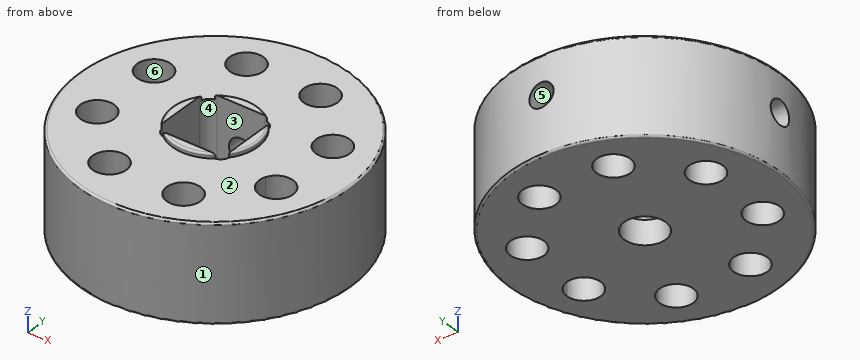
```python
from build123d import *

# Parameters (mm, degrees)
F0_R          = 14
F1_DEPTH      = 10
F2_R          = 4.4
F3_DEPTH      = 0.5
F4_W          = 7
F4_H          = 7
F5_DEPTH      = 8
F6_R          = 2.15
F7_DEPTH      = 2.5
F8_R          = 1.75
F9_DEPTH      = 10
F10_R         = 1.25
F11_DEPTH     = 25
F12_R         = 1.25
F13_DEPTH     = 25
F14_T1_DEPTH  = 10
F14_T6_DEPTH  = 12.5
F14_S7_R      = 4.4
F14_T8_DEPTH  = 8
F14_T13_DEPTH = 12.5
F14_S14_R     = 4.4
F14_T15_DEPTH = 8
F14_T20_DEPTH = 12.5
F14_S21_R     = 4.4
F14_T22_DEPTH = 8
F14_T27_DEPTH = 12.5
F14_S28_R     = 4.4
F14_T29_DEPTH = 8
F15_R         = 0.2


# Not quite as in the source:
# - a fillet or chamfer that OpenCascade refuses, or shapes differently, is made with other operations: its cross-section is extruded or revolved along the edge and cut away or added
# - a feature names something its author has since deleted; it is built from what else it names


with BuildPart() as f1:
    # F0 (on Top) → F1 (new body)
    with BuildSketch(Plane.XY):
        Circle(F0_R)
    extrude(amount=F1_DEPTH)

    # F2 (on face) → F3 (join)
    with BuildSketch(Plane.XY.offset(10)):
        Circle(F2_R)
    extrude(amount=F3_DEPTH)

    # F4 (on face) → F5 (cut)
    with BuildSketch(Plane.XY.offset(10.5)):
        Rectangle(F4_W, F4_H)
    extrude(amount=-F5_DEPTH, mode=Mode.SUBTRACT)

    # F6 (on face) → F7 (cut, through all)
    with BuildSketch(Plane(origin=(0, 0, 0), x_dir=(1, 0, 0), z_dir=(0, 0, -1))):
        Circle(F6_R)
    extrude(amount=-F7_DEPTH, mode=Mode.SUBTRACT)

    # F8 (on face) → F9 (cut, through all)
    with BuildSketch(Plane(origin=(0, 0, 0), x_dir=(1, 0, 0), z_dir=(0, 0, -1))):
        with BuildLine():
            ThreePointArc((7.6220061432, 3.157138317), (9.5802033886, 2.1104600829), (10.9887953251, 3.8268343237))
            ThreePointArc((10.9887953251, 3.8268343237), (8.8973872616, 5.5432085644), (7.6220061432, 3.157138317))
        make_face()
        with Locations((3.8268343237, 9.2387953251)):
            Circle(F8_R)
        with Locations((-3.8268343237, 9.2387953251)):
            Circle(F8_R)
        with Locations((-9.2387953251, 3.8268343237)):
            Circle(F8_R)
        with Locations((-9.2387953251, -3.8268343237)):
            Circle(F8_R)
        with Locations((-3.8268343237, -9.2387953251)):
            Circle(F8_R)
        with Locations((3.8268343237, -9.2387953251)):
            Circle(F8_R)
        with Locations((9.2387953251, -3.8268343237)):
            Circle(F8_R)
    extrude(amount=-F9_DEPTH, mode=Mode.SUBTRACT)

    # F10 (on Front) → F11 (cut)
    with BuildSketch(Plane.XZ):
        with Locations((0, 6)):
            Circle(F10_R)
    extrude(amount=-F11_DEPTH, mode=Mode.SUBTRACT)

    # F12 (on Right) → F13 (cut)
    with BuildSketch(Plane.YZ):
        with Locations((0, 6)):
            Circle(F12_R)
    extrude(amount=-F13_DEPTH, mode=Mode.SUBTRACT)

    # F14: fillet of radius 1 on 4 edges, made by hand

    # F14_s2 → F14_t1 (join)
    with BuildSketch(Plane.XY):
        with BuildLine():
            ThreePointArc((-2.5, -3.5), (-3.2071067812, -3.2071067812), (-3.5, -2.5))
            Line((-3.5, -2.5), (-3.5, -3.5))
            Line((-3.5, -3.5), (-2.5, -3.5))
        make_face()
        with BuildLine():
            ThreePointArc((3.5, -2.5), (3.2071067812, -3.2071067812), (2.5, -3.5))
            Line((2.5, -3.5), (3.5, -3.5))
            Line((3.5, -3.5), (3.5, -2.5))
        make_face()
        with BuildLine():
            ThreePointArc((3.5, 2.5), (3.2071067812, 3.2071067812), (2.5, 3.5))
            Line((2.5, 3.5), (3.5, 3.5))
            Line((3.5, 3.5), (3.5, 2.5))
        make_face()
        with BuildLine():
            ThreePointArc((-2.5, 3.5), (-3.2071067812, 3.2071067812), (-3.5, 2.5))
            Line((-3.5, 2.5), (-3.5, 3.5))
            Line((-3.5, 3.5), (-2.5, 3.5))
        make_face()
    extrude(amount=F14_T1_DEPTH)


with BuildPart() as f14_tool4:
    # F14_s5 → F14_t6 (new body)
    with BuildSketch(Plane.XY.offset(12.5)):
        with BuildLine():
            ThreePointArc((-2.5, -3.5), (-3.2071067812, -3.2071067812), (-3.5, -2.5))
            Line((-3.5, -2.5), (-3.5, -3.5))
            Line((-3.5, -3.5), (-2.5, -3.5))
        make_face()
    extrude(amount=-F14_T6_DEPTH)

    # F14_s7 → F14_t8 (intersect, symmetric)
    with BuildSketch(Plane.XY.offset(6.2)):
        Circle(F14_S7_R)
    extrude(amount=F14_T8_DEPTH, both=True, mode=Mode.INTERSECT)

    split(bisect_by=Plane.XY.offset(10.5), keep=Keep.BOTTOM)


with BuildPart() as f1_1:
    add(f1.part)

    # F14_t3: union F14_tool4
    add(f14_tool4.part)


with BuildPart() as f14_tool11:
    # F14_s12 → F14_t13 (new body)
    with BuildSketch(Plane.XY.offset(12.5)):
        with BuildLine():
            ThreePointArc((3.5, -2.5), (3.2071067812, -3.2071067812), (2.5, -3.5))
            Line((2.5, -3.5), (3.5, -3.5))
            Line((3.5, -3.5), (3.5, -2.5))
        make_face()
    extrude(amount=-F14_T13_DEPTH)

    # F14_s14 → F14_t15 (intersect, symmetric)
    with BuildSketch(Plane.XY.offset(6.2)):
        Circle(F14_S14_R)
    extrude(amount=F14_T15_DEPTH, both=True, mode=Mode.INTERSECT)

    split(bisect_by=Plane.XY.offset(10.5), keep=Keep.BOTTOM)


with BuildPart() as f1_2:
    add(f1_1.part)

    # F14_t10: union F14_tool11
    add(f14_tool11.part)


with BuildPart() as f14_tool18:
    # F14_s19 → F14_t20 (new body)
    with BuildSketch(Plane.XY.offset(12.5)):
        with BuildLine():
            ThreePointArc((3.5, 2.5), (3.2071067812, 3.2071067812), (2.5, 3.5))
            Line((2.5, 3.5), (3.5, 3.5))
            Line((3.5, 3.5), (3.5, 2.5))
        make_face()
    extrude(amount=-F14_T20_DEPTH)

    # F14_s21 → F14_t22 (intersect, symmetric)
    with BuildSketch(Plane.XY.offset(6.2)):
        Circle(F14_S21_R)
    extrude(amount=F14_T22_DEPTH, both=True, mode=Mode.INTERSECT)

    split(bisect_by=Plane.XY.offset(10.5), keep=Keep.BOTTOM)


with BuildPart() as f1_3:
    add(f1_2.part)

    # F14_t17: union F14_tool18
    add(f14_tool18.part)


with BuildPart() as f14_tool25:
    # F14_s26 → F14_t27 (new body)
    with BuildSketch(Plane.XY.offset(12.5)):
        with BuildLine():
            ThreePointArc((-2.5, 3.5), (-3.2071067812, 3.2071067812), (-3.5, 2.5))
            Line((-3.5, 2.5), (-3.5, 3.5))
            Line((-3.5, 3.5), (-2.5, 3.5))
        make_face()
    extrude(amount=-F14_T27_DEPTH)

    # F14_s28 → F14_t29 (intersect, symmetric)
    with BuildSketch(Plane.XY.offset(6.2)):
        Circle(F14_S28_R)
    extrude(amount=F14_T29_DEPTH, both=True, mode=Mode.INTERSECT)

    split(bisect_by=Plane.XY.offset(10.5), keep=Keep.BOTTOM)


with BuildPart() as f1_4:
    add(f1_3.part)

    # F14_t24: union F14_tool25
    add(f14_tool25.part)

    # F15
    f15_edges = [f1_4.edges().sort_by_distance(p)[0] for p in [
        (-14, 0, 10),
        (-14, 0, 0),
        (-4.4, 0, 10.5),
        (0, -4.4, 10.5),
        (4.4, 0, 10.5),
        (0, 4.4, 10.5),
    ]]
    fillet(f15_edges, radius=F15_R)


solid = f1_4.part
```
CAD build for the part. Positions are in the model's coordinates, mm. Face numbers are marked on the shaded views. A direction names the side the tool comes from. Coordinates: 2 decimals unless noted, no trailing zeros. Write each loop counter-clockwise with the first axis right and the second up, starting at its lowest first coordinate (ties: lowest second). Pieces come first, ordered by that corner, then holes. Notation, with made-up numbers: (54.25, 46.5) -> (68.25, 46.5) arc R19 ccw to (68.25, 56.5) -> close; hole circle Ø1 at (23.5, -34). An arc over 180 degrees is marked (long way). Return JSON: item names as keys, results as strings. Group by question number.
Q1. Cut at B-B, the plane x = 0. Give the cut face in (y, z).
Q2. Cut at A-A, the plane y = 0. Give the cut face in (x, z), then the cut area to 3 significant figures.
Q3. Which spindle directions (+Z, -Z, +X, -X, +Y, -Y) get a long thin tool onto all of the face, cutting with end or side? Do the marked faces 4, 5 and 6. Say none if no direction does.
Q4. Pull direction X, two halves, no side cores. Call the marked faces 1, 2 and 3: released by +X, released by -X, zero draft, split by the parting line, or undercut.
Q5. Drill centre lines: line 1 (Z direction, x = 0, y = 11.75); line 2 (Y direction, x = -8, z = 1.5). Where is each one in solid material? Low to high.
Q6. Flat gauge pins, fed straight in: pin 1 (4.5 mm diameter, centred on x = 9.24, y = -3.83, fed in from -Z); pin 2 (1.5 mm diameter, centred on x = -5.5, z = 8.5, fed in from +Y); pin 3 (4 mm diameter, centred on y = 8.5, z = 2.5, fed in from -X); pin 4 (4 mm diameter, centred on x = 3.83, y = 9.24, fed in from +Z). Where does each tip first touch, or does it go through?
Q7. Cut at C-C, the plane z = 6.75. State how many separate pieces and enclosed holes the cut face has, then the cut area to 3 significant figures.
Returned:
{
 "1": {"outline": "(-14, 0.2) arc R0.2 ccw to (-13.8, 0) -> (-2.15, 0) -> (-2.15, 2.5) -> (-3.5, 2.5) -> (-3.5, 10.5) -> (-4.2, 10.5) arc R0.2 ccw to (-4.4, 10.3) -> (-4.4, 10) -> (-13.8, 10) arc R0.2 ccw to (-14, 9.8) -> close; (2.15, 0) -> (13.8, 0) arc R0.2 ccw to (14, 0.2) -> (14, 4.75) -> (3.5, 4.75) -> (3.5, 2.5) -> (2.15, 2.5) -> close; (3.5, 7.25) -> (14, 7.25) -> (14, 9.8) arc R0.2 ccw to (13.8, 10) -> (4.4, 10) -> (4.4, 10.3) arc R0.2 ccw to (4.2, 10.5) -> (3.5, 10.5) -> close"},
 "2": {"outline": "(-14, 0.2) arc R0.2 ccw to (-13.8, 0) -> (-2.15, 0) -> (-2.15, 2.5) -> (-3.5, 2.5) -> (-3.5, 4.75) -> (-14, 4.75) -> close; (-14, 7.25) -> (-3.5, 7.25) -> (-3.5, 10.5) -> (-4.2, 10.5) arc R0.2 ccw to (-4.4, 10.3) -> (-4.4, 10) -> (-13.8, 10) arc R0.2 ccw to (-14, 9.8) -> close; (2.15, 0) -> (13.8, 0) arc R0.2 ccw to (14, 0.2) -> (14, 9.8) arc R0.2 ccw to (13.8, 10) -> (4.4, 10) -> (4.4, 10.3) arc R0.2 ccw to (4.2, 10.5) -> (3.5, 10.5) -> (3.5, 2.5) -> (2.15, 2.5) -> close", "area": "191 mm2"},
 "3": {"face 4": "+Z", "face 5": "+Y", "face 6": "+Z, -Z"},
 "4": {"face 1": "split by the parting line", "face 2": "zero draft", "face 3": "undercut"},
 "5": {"line 1": "z = 0 to 4.75, 7.25 to 10", "line 2": "y = -11.49 to -5.06, -2.59 to 2.59, 5.06 to 11.49"},
 "6": {"pin 1": "stops at z = 0", "pin 2": "stops at y = 13.17", "pin 3": "stops at x = -12.4", "pin 4": "stops at z = 10"},
 "7": {"separate pieces": "2", "enclosed holes": "8", "area": "449 mm2"}
}
